CAD build for the part. Positions are in the model's coordinates, mm. Face numbers are marked on the shaded views. A direction names the side the tool comes from. Give positions to 0.01 mm unless a question says otherwise; leave off trailing zeros. Loops run counter-clockwise (first coordinate to the right, second up) from the corner with the lowest first, then second, coordinate; pieces in that order, holes last.
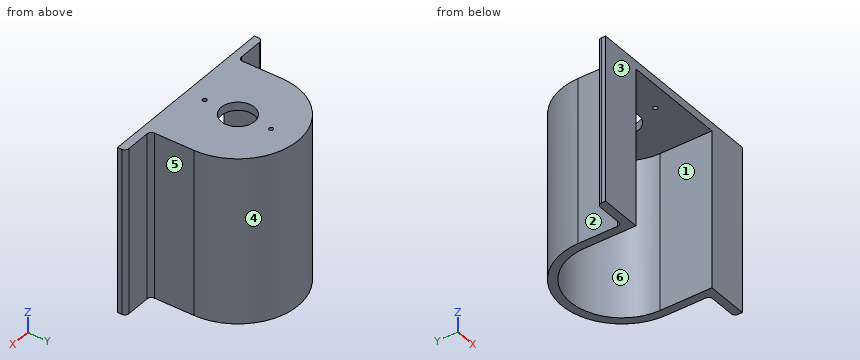
```python
from build123d import *

# Parameters (mm, degrees)
BOSS_EXTRU_1_DEPTH      = 40
ESQUISSE2_W             = 2
ESQUISSE2_H             = 40
BOSS_EXTRU_2_DEPTH      = 12.5
ESQUISSE3_W             = 10
ESQUISSE3_H             = 40
BOSS_EXTRU_3_DEPTH      = 2
BOSS_EXTRU_4_START      = -2
ESQUISSE4_R             = 4
BOSS_EXTRU_4_DEPTH      = 2
CONG_1_R                = 1
ESQUISSE5_R             = 0.5
ENL_V_MAT_EXTRU_1_DEPTH = 49.130032204


with BuildPart() as part:
    # Esquisse1 → Boss.-Extru.1 (new body)
    with BuildSketch(Plane.XY):
        with BuildLine():
            ThreePointArc((-12.5, 0), (0, 12.5), (12.5, 0))
            Line((12.5, 0), (14.5, 0))
            ThreePointArc((14.5, 0), (0, 14.5), (-14.5, 0))
            Line((-14.5, 0), (-12.5, 0))
        make_face()
    extrude(amount=BOSS_EXTRU_1_DEPTH)

    # Esquisse2 → Boss.-Extru.2 (add)
    with BuildSketch(Plane.XZ):
        with Locations((-13.5, 20)):
            Rectangle(ESQUISSE2_W, ESQUISSE2_H)
        with Locations((13.5, 20)):
            Rectangle(ESQUISSE2_W, ESQUISSE2_H)
    extrude(amount=BOSS_EXTRU_2_DEPTH)

    # Esquisse3 → Boss.-Extru.3 (add)
    with BuildSketch(Plane.XZ.offset(12.5)):
        with Locations((-17.5, 20)):
            Rectangle(ESQUISSE3_W, ESQUISSE3_H)
        with Locations((17.5, 20)):
            Rectangle(ESQUISSE3_W, ESQUISSE3_H)
    extrude(amount=-BOSS_EXTRU_3_DEPTH)

    # Esquisse4 → Boss.-Extru.4 (add)
    with BuildSketch(Plane.XY.offset(40).offset(BOSS_EXTRU_4_START)):
        with BuildLine():
            Line((-12.5, 0), (-12.5, -12.5))
            Line((-12.5, -12.5), (12.5, -12.5))
            Line((12.5, -12.5), (12.5, 0))
            ThreePointArc((12.5, 0), (0, 12.5), (-12.5, 0))
        make_face()
        Circle(ESQUISSE4_R, mode=Mode.SUBTRACT)
    extrude(amount=BOSS_EXTRU_4_DEPTH)

    # Congé1
    cong_1_edges = [part.edges().sort_by_distance(p)[0] for p in [
        (-22.5, -10.5, 20),
        (-14.5, -10.5, 20),
        (14.5, -10.5, 20),
        (22.5, -10.5, 20),
    ]]
    fillet(cong_1_edges, radius=CONG_1_R)

    # Esquisse5 → Enlèv. mat.-Extru.1 (cut, through all)
    with BuildSketch(Plane.XY.offset(40)):
        with Locations((0, -8)):
            Circle(ESQUISSE5_R)
        with Locations((0, 8)):
            Circle(ESQUISSE5_R)
    extrude(amount=-ENL_V_MAT_EXTRU_1_DEPTH, mode=Mode.SUBTRACT)


solid = part.part
```
1. Tool access for the marked faces 4, 5 and 6: list every direction of +Z, -Z, +X, -X, +Y, -Y with a clear straight run to the whole face (end or side of a thin tool).
Responses:
face 4: +Z, -Z, +Y
face 5: +Z, -Z, +X, +Y
face 6: -Z, -Y
2. Pull direction X, two halves, no side cores. Call the marked faces 1, 2 and 3: released by +X, released by -X, zero draft, split by the parting line, or undercut.
Responses:
face 1: undercut
face 2: released by -X
face 3: zero draft
3. Probe line 1 along Y through (x, z) = (0, 38.65); line 2 along X through (y, z) = (-5.75, 36.5); line 3 along Z through (x, y) = (11.5, 1.5). List the from-to ranges inside material, lowest first.
Responses:
line 1: y = -12.5 to -8.5, -7.5 to -4, 4 to 7.5, 8.5 to 14.5
line 2: x = -14.5 to -12.5, 12.5 to 14.5
line 3: z = 38 to 40
4. Saw through at A-A, the plane x = 2. List the corners of the cut face in (y, z).
Responses:
outline: (-12.5, 38) - (-3.46, 38) - (-3.46, 40) - (-12.5, 40) - close; (3.46, 38) - (12.34, 38) - (12.34, 0) - (14.36, 0) - (14.36, 40) - (3.46, 40) - close
5. Saw through at D-D, the plane x = 17.5. List the corners of the cut face in (y, z).
Responses:
outline: (-12.5, 0) - (-10.5, 0) - (-10.5, 40) - (-12.5, 40) - close
6. Drop flat-ended pins along their axis: pin 1 (10 mm diameter, centred on x = 18, y = -6, fed in from +Z); pin 2 (2 mm diameter, centred on y = 1, z = 21, fed in from +X); pin 3 (1.5 mm diameter, centred on x = 1, y = -3.5, fed in from -Z); pin 4 (5 mm diameter, centred on x = -17.5, z = 12, fed in from +Y). Give the stop position or say it passes through.
Responses:
pin 1: stops at z = 40
pin 2: stops at x = 14.5
pin 3: stops at z = 38
pin 4: stops at y = -10.37
7. Saw through at B-B, the plane z = 14.5. List the corners of the cut face in (x, y).
Responses:
outline: (-22.5, -12.5) - (-12.5, -12.5) - (-12.5, 0) arc R12.5 cw to (12.5, 0) - (12.5, -12.5) - (22.5, -12.5) - (22.5, -11.5) arc R1 ccw to (21.5, -10.5) - (15.5, -10.5) arc R1 cw to (14.5, -9.5) - (14.5, 0) arc R14.5 ccw to (-14.5, 0) - (-14.5, -9.5) arc R1 cw to (-15.5, -10.5) - (-21.5, -10.5) arc R1 ccw to (-22.5, -11.5) - close
8. Saw through at C-C, the plane y = 6. List the corners of the cut face in (x, z).
Responses:
outline: (-13.2, 0) - (-10.97, 0) - (-10.97, 38) - (10.97, 38) - (10.97, 0) - (13.2, 0) - (13.2, 40) - (-13.2, 40) - close
